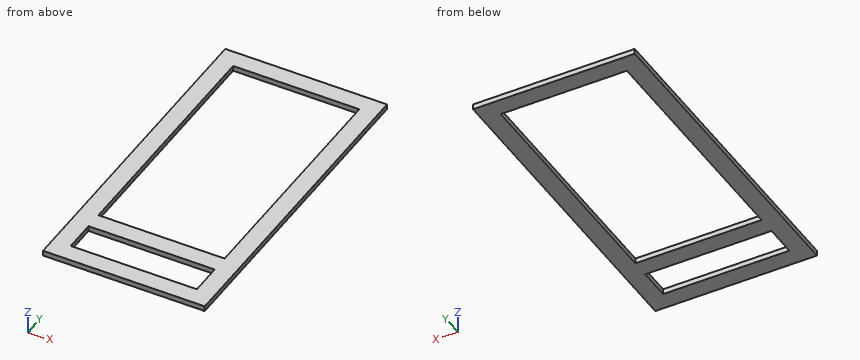
from build123d import *

# Parameters (mm, degrees)
CROQUIS1_W              = 454.7
CROQUIS1_H              = 920
CROQUIS1_W_2            = 354.7
CROQUIS1_H_2            = 680
SALIENTE_EXTRUIR1_DEPTH = 15
CROQUIS2_W              = 354.7
CROQUIS2_H              = 90
CORTAR_EXTRUIR1_DEPTH   = 15


with BuildPart() as part:
    # Croquis1 → Saliente-Extruir1 (new body)
    with BuildSketch(Plane.XY):
        Rectangle(CROQUIS1_W, CROQUIS1_H)
        with Locations((0, 70)):
            Rectangle(CROQUIS1_W_2, CROQUIS1_H_2, mode=Mode.SUBTRACT)
    extrude(amount=-SALIENTE_EXTRUIR1_DEPTH)

    # Croquis2 → Cortar-Extruir1 (cut)
    with BuildSketch(Plane.XY):
        with Locations((0, -365)):
            Rectangle(CROQUIS2_W, CROQUIS2_H)
    extrude(amount=-CORTAR_EXTRUIR1_DEPTH, mode=Mode.SUBTRACT)


solid = part.part
Design review of the part built by this model. Coordinates are the model's own, in mm. Give positions to 0.01 mm unless a question says otherwise; leave off trailing zeros. Order: outer loops, then holes, each group sorted by start corner. A loop starts at its lowest first (then second) coordinate and runs counter-clockwise, first axis right, second up. Notation, with made-up numbers: (79, -26) - (96, -26) arc R26 cw to (96, 2) - close; hole circle Ø11 at (18.25, 22.25). An arc over 180 degrees is marked (long way). Write item = value, one per line. Start each with the question number.
Q1. We need section B-B on y = 220.5. State the section outline as (x, z) points.
Q2. We need section C-C on x = -3. State the section outline as (y, z) points, plus the area to 3 significant figures.
Q3. To check wall thickness, follow L1, parallel to Y at x = 122.5, z = -3.75; L2, parallel to X at y = -159.5, z = -1.75. State the ranges of each line that lie inside material, in increasing order. Write a range as from..to.
Q4. We need section A-A on z = -5.5. State the section outline as (x, y) points, plus the area to 3 significant figures.
Working result:
q1.outline = (-227.35, -15) - (-177.35, -15) - (-177.35, 0) - (-227.35, 0) - close; (177.35, -15) - (227.35, -15) - (227.35, 0) - (177.35, 0) - close
q2.outline = (-460, -15) - (-410, -15) - (-410, 0) - (-460, 0) - close; (-320, -15) - (-270, -15) - (-270, 0) - (-320, 0) - close; (410, -15) - (460, -15) - (460, 0) - (410, 0) - close
q2.area = 2,250 mm²
q3.L1 = -460..-410, -320..-270, 410..460
q3.L2 = -227.35..-177.35, 177.35..227.35
q4.outline = (-227.35, -460) - (227.35, -460) - (227.35, 460) - (-227.35, 460) - close; hole (-177.35, -410) - (177.35, -410) - (177.35, -320) - (-177.35, -320) - close; hole (-177.35, -270) - (177.35, -270) - (177.35, 410) - (-177.35, 410) - close
q4.area = 145,000 mm²
